```python
from build123d import *

# Parameters (mm, degrees)
SKETCH1_R                = 3.1
BOSS_EXTRUDE1_DEPTH      = 35
SKETCH2_R                = 3.1
BOSS_EXTRUDE2_DEPTH      = 20
BOSS_EXTRUDE3_DEPTH      = 35
SKETCH4_R                = 2.6
CUT_EXTRUDE1_DEPTH       = 59.014006929
SKETCH6_W                = 12.5
SKETCH6_H                = 8
CUT_EXTRUDE2_DEPTH       = 58.241265709
SKETCH7_W                = 48
SKETCH7_H                = 35
BOSS_EXTRUDE4_DEPTH      = 10
SKETCH8_W                = 14
SKETCH8_H                = 35
SKETCH8_R                = 3.1
BOSS_EXTRUDE5_DEPTH      = 5
BOSS_EXTRUDE6_DEPTH      = 2.4
BOSS_EXTRUDE6_DEPTH_BACK = 4.85
SKETCH9_R                = 1.2
CHAMFER1_SIZE            = 2


with BuildPart() as part:
    # Sketch1 → Boss-Extrude1 (new body)
    with BuildSketch(Plane.XY):
        Polygon((-5, -3.75), (-35, -3.75), (-35, -28.75), (13, -28.75), (13, -3.75), align=None)
        with Locations((5, -15.75)):
            Circle(SKETCH1_R, mode=Mode.SUBTRACT)
        with Locations((-27, -15.75)):
            Circle(SKETCH1_R, mode=Mode.SUBTRACT)
    extrude(amount=BOSS_EXTRUDE1_DEPTH)

    # Sketch2 → Boss-Extrude2 (add)
    with BuildSketch(Plane(origin=(0, 0, 0), x_dir=(-1, 0, 0), z_dir=(0, 0, -1))):
        with Locations((27, -15.75)):
            Circle(SKETCH2_R)
        with Locations((-5, -15.75)):
            Circle(SKETCH2_R)
    extrude(amount=-BOSS_EXTRUDE2_DEPTH)

    # Sketch3 → Boss-Extrude3 (add)
    with BuildSketch(Plane.XY.offset(35)):
        Polygon((-17.25, 2.5), (-17.25, -7.5), (-23.25, -7.5), (-23.25, 12.5), (-17.25, 12.5), align=None)
        Polygon((-4.75, 2.5), (-4.75, -7.5), (1.25, -7.5), (1.25, 12.5), (-4.75, 12.5), align=None)
    extrude(amount=-BOSS_EXTRUDE3_DEPTH)

    # Sketch4 → Cut-Extrude1 (cut, through all)
    with BuildSketch(Plane.ZY.offset(23.25)):
        with Locations((17.5, 2.5)):
            Circle(SKETCH4_R)
        with Locations((27.5, 2.5)):
            Circle(SKETCH4_R)
        with Locations((7.5, 2.5)):
            Circle(SKETCH4_R)
    extrude(amount=-CUT_EXTRUDE1_DEPTH, mode=Mode.SUBTRACT)

    # Sketch6 → Cut-Extrude2 (cut, through all)
    with BuildSketch(Plane.XY.offset(35)):
        with Locations((-11, -7.75)):
            Rectangle(SKETCH6_W, SKETCH6_H)
    extrude(amount=-CUT_EXTRUDE2_DEPTH, mode=Mode.SUBTRACT)

    # Sketch7 → Boss-Extrude4 (add)
    with BuildSketch(Plane.XZ.offset(28.75)):
        with Locations((-11, 17.5)):
            Rectangle(SKETCH7_W, SKETCH7_H)
    extrude(amount=BOSS_EXTRUDE4_DEPTH)

    # Sketch8 → Boss-Extrude5 (add)
    # profile 1 of 2: a face of its own
    with BuildSketch(Plane.XZ.offset(38.75)):
        with Locations((-42, 17.5)):
            Rectangle(SKETCH8_W, SKETCH8_H)
        with Locations(Location((-42, 9, 0), (0, 0, 270))):
            Circle(SKETCH8_R, mode=Mode.SUBTRACT)
        with Locations(Location((-42, 26, 0), (0, 0, 270))):
            Circle(SKETCH8_R, mode=Mode.SUBTRACT)
    # profile 2 of 2: a face of its own
    with BuildSketch(Plane.XZ.offset(38.75)):
        with Locations((20, 17.5)):
            Rectangle(SKETCH8_W, SKETCH8_H)
        with Locations(Location((20, 9, 0), (0, 0, 90))):
            Circle(SKETCH8_R, mode=Mode.SUBTRACT)
        with Locations(Location((20, 26, 0), (0, 0, 270))):
            Circle(SKETCH8_R, mode=Mode.SUBTRACT)
    extrude(amount=-BOSS_EXTRUDE5_DEPTH)

    # Sketch9 → Boss-Extrude6 (add, two sides: drawn at the far end of the back side and taken through both)
    with BuildSketch(Plane(origin=(-30.15, 41.369079409, 256.718616892), x_dir=(0, 0, -1), z_dir=(1, 0, 0)).offset(-BOSS_EXTRUDE6_DEPTH_BACK)):
        Polygon((230.018616892, -24.119079409), (230.018616892, -45.119079409), (230.018616892, -49.119079409), (221.718616892, -49.119079409), (221.718616892, -24.119079409), align=None)
        with Locations(Location((225.868616892, -29.469079409, 0), (0, 0, 90))):
            Circle(SKETCH9_R, mode=Mode.SUBTRACT)
        with Locations(Location((225.868616892, -39.069079409, 0), (0, 0, 90))):
            Circle(SKETCH9_R, mode=Mode.SUBTRACT)
    extrude(amount=BOSS_EXTRUDE6_DEPTH + BOSS_EXTRUDE6_DEPTH_BACK)

    # Chamfer1
    chamfer1_edges = [part.edges().sort_by_distance(p)[0] for p in [
        (-27.75, -3.75, 30.85),
        (-31.375, -3.75, 26.7),
    ]]
    chamfer(chamfer1_edges, length=CHAMFER1_SIZE)


solid = part.part
```
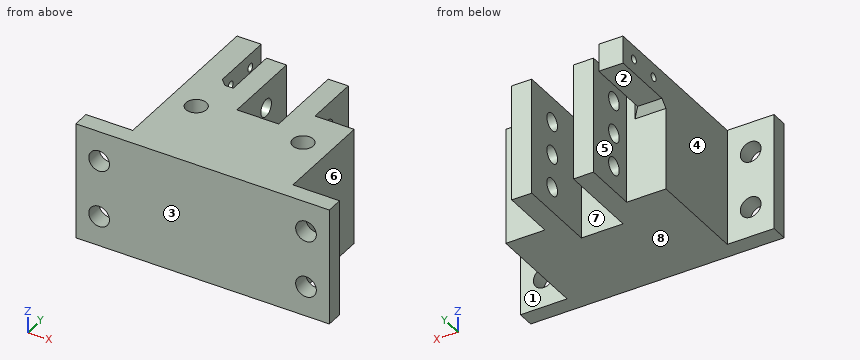
Can you work these out from the model? Positions are in its coordinate system, mm. Face numbers are marked on the shaded views. A direction names the side the tool comes from. Round coordinates to 2 decimals unless told otherwise and drop trailing zeros. Loops run counter-clockwise (first coordinate to the right, second up) from the corner with the lowest first, then second, coordinate; pieces in that order, holes last. Notation, with made-up numbers: (-40, -7.5) -> (-12, -7.5) arc R29 ccw to (-12, 30.5) -> close; hole circle Ø4 at (69.5, -3). An arc over 180 degrees is marked (long way). One line per item, written item: value. Start each with the question number.
1. If we section it at B-B, the plane y = 6: Write out the boundary of the cut face in (x, z), then the cut area to 3 significant figures.
2. For pin 1 (3 mm diameter, centred on x = 4, y = -16.5, fed in from +Z); pin 2 (12 mm diameter, centred on y = -14, z = 3.5, fed in from +X); pin 3 (7 mm diameter, centred on x = 20, z = 17, fed in from +Y); pin 4 (5.5 mm diameter, centred on x = -42, z = 26, fed in from -Y), each with a flat end and sliding along its axis, tell me the tip position at first contact or that it passes through.
3. If I drill on probe 1 along X at (y, z) = (-35, 9); probe 2 along X at (y, z) = (-6, 16); probe 3 along Z at (x, y) = (19.5, -36), over which ranges is the centre line in solid material (lowest first)?
4. For the marked faces 1, 2, 3, 4 and 5, which set-ups out of +Z, -Z, +X, -X, +Y, -Y let a thin tool reach every point of the face, with its end or its side?
5. If we mould it in two halves opening along X, with no side actions, what happens to the marked faces 6, 7 and 8? For each: pulls with the +X half, pulls with the -X half, needs draft (parallel to the pull), parting line crosses it, or undercut.
6. If we section it at C-C, the plane z = 9: Give the number of separate pieces and of enclosed holes in the cut face, then the cut area to 3 significant figures.
7. If we section it at D-D, the plane z = 21.5: Write out the boundary of the cut face in (x, y).
8. If we section it at A-A, the plane x = -42: Write out the boundary of the cut face in (y, z).
Calculated:
1. outline: (-35, 26.7) -> (-27.75, 26.7) -> (-27.75, 35) -> (-35, 35) -> close; (-23.25, 0) -> (-17.25, 0) -> (-17.25, 35) -> (-23.25, 35) -> close; (-4.75, 0) -> (1.25, 0) -> (1.25, 35) -> (-4.75, 35) -> close
1. area: 480 mm²
2. pin 1: stops at z = 20
2. pin 2: stops at x = 13
2. pin 3: stops at y = -33.75
2. pin 4: passes through
3. probe 1: x = -49 to -45.1, -38.9 to 16.9, 23.1 to 27
3. probe 2: x = -35 to -17.25, -4.75 to 13
3. probe 3: z = 0 to 5.94, 12.06 to 22.94, 29.06 to 35
4. face 1: +Z, -Z, +X, +Y
4. face 2: -Z, -X, +Y
4. face 3: +Z, -Z, +X, -X, -Y
4. face 4: +Z, -Z, -X, +Y
4. face 5: +Z, -Z, +Y
5. face 6: pulls with the +X half
5. face 7: undercut
5. face 8: needs draft
6. separate pieces: 5
6. enclosed holes: 0
6. area: 1,800 mm²
7. outline: (-49, -38.75) -> (27, -38.75) -> (27, -33.75) -> (13, -33.75) -> (13, -3.75) -> (1.25, -3.75) -> (1.25, 12.5) -> (-4.75, 12.5) -> (-4.75, -11.75) -> (-17.25, -11.75) -> (-17.25, 12.5) -> (-23.25, 12.5) -> (-23.25, -3.75) -> (-35, -3.75) -> (-35, -33.75) -> (-49, -33.75) -> close; hole circle Ø6.2 at (-27, -15.75); hole circle Ø6.2 at (5, -15.75)
8. outline: (-38.75, 0) -> (-33.75, 0) -> (-33.75, 5.9) -> (-38.75, 5.9) -> close; (-38.75, 12.1) -> (-33.75, 12.1) -> (-33.75, 22.9) -> (-38.75, 22.9) -> close; (-38.75, 29.1) -> (-33.75, 29.1) -> (-33.75, 35) -> (-38.75, 35) -> close
